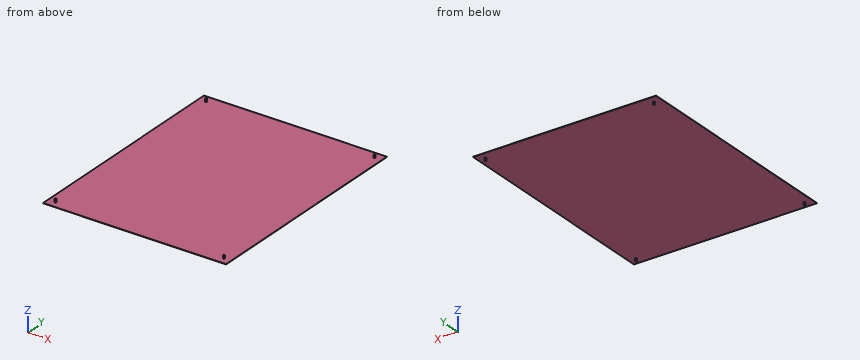
from build123d import *

# Parameters (mm, degrees)
SKETCH1_W           = 635
SKETCH1_H           = 789.432
BOSS_EXTRUDE1_DEPTH = 0.999998
SKETCH2_R           = 3.175
BOSS_EXTRUDE2_DEPTH = 9.525


with BuildPart() as part:
    # Sketch1 → Boss-Extrude1 (new body)
    with BuildSketch(Plane.XY):
        Rectangle(SKETCH1_W, SKETCH1_H)
    extrude(amount=BOSS_EXTRUDE1_DEPTH)

    # Sketch2 → Boss-Extrude2 (add, symmetric)
    with BuildSketch(Plane.XY.offset(0.999998)):
        with Locations(Location((-292.1, 369.316, 0), (0, 0, 180))):
            Circle(SKETCH2_R)
        with Locations(Location((292.1, 369.316, 0), (0, 0, 180))):
            Circle(SKETCH2_R)
        with Locations(Location((-292.1, -369.316, 0), (0, 0, 180))):
            Circle(SKETCH2_R)
        with Locations(Location((292.1, -369.316, 0), (0, 0, 180))):
            Circle(SKETCH2_R)
    extrude(amount=BOSS_EXTRUDE2_DEPTH, both=True)


solid = part.part
Source: CAD feature listing. Evaluate the final solid. Frame: model axes, mm. Round coordinates to 2 decimals unless told otherwise and drop trailing zeros. Write each loop counter-clockwise with the first axis right and the second up, starting at its lowest first coordinate (ties: lowest second). Pieces come first, ordered by that corner, then holes. Notation, with made-up numbers: (88, 72) - (129, 72) arc R9 cw to (129, 83) - close; hole circle Ø5 at (-36.5, 15). An arc over 180 degrees is marked (long way). Use CSV: the item, a comma, the result in double quotes. Start each with the question number.
(1) Cut plane B-B, the plane x = 262. Return loops of the section in (y, z), and give its area (3 significant figures).
(2) Cut plane A-A, the plane y = 56.5. Return loops of the section in (x, z).
(3) First-contact query: pin 1 Ø4 at (x, y) = (250, -210) entering from -Z; pin 2 Ø4 at (x, y) = (-87.5, 76.5) entering from +Z. Flat tips, straight axial feed; report the tip coordinate or a pass-through.
(4) Cut plane C-C, the plane z = -5.25. Return loops of the section in (x, y) (3 decimals).
(5) Material intervals for probe 1 along Z at (x, y) = (64, 158.5), sorted ascending. Write a range as [from, to].
Geometry says:
1,outline,"(-394.72, 0) - (394.72, 0) - (394.72, 1) - (-394.72, 1) - close"
1,area,"789 mm²"
2,outline,"(-317.5, 0) - (317.5, 0) - (317.5, 1) - (-317.5, 1) - close"
3,pin 1,"z = 0"
3,pin 2,"z = 1"
4,outline,"circle Ø6.35 at (-292.1, -369.316); circle Ø6.35 at (-292.1, 369.316); circle Ø6.35 at (292.1, -369.316); circle Ø6.35 at (292.1, 369.316)"
5,probe 1,"[0, 1]"
